Could you check a few things on this model? Use its own coordinates, in mm. Coordinates: 2 decimals unless noted, no trailing zeros. Answer as CSV lines item,"result". Start each with the question number.
Item 1: Suppose I cut it at A-A, the plane z = 378. State how many separate pieces and enclosed holes the cut face has, and give its area (3 significant figures).
Item 2: I'm going to push flat-ended pins straight in: P1, Ø2.5, axis at y = -1.5, z = 150.5, coming from the +X side; P2, Ø1.5, axis at x = -10.5, z = 110.5, coming from the -Y side. Where does each tip first touch, or does it pass through?
Item 3: If I drill on line 1 along X through (y, z) = (7, 64.5); line 2 along Y through (x, z) = (-15, 459); line 3 along Y through (x, z) = (-9.5, 274), over which ranges is the centre line in solid material (lowest first)? Write a range as [from, to].
```python
from build123d import *

# Parameters (mm, degrees)
F0_R     = 2.1
F1_DEPTH = 500


with BuildPart() as f1:
    # F0 (on Top) → F1 (new body)
    with BuildSketch(Plane.XY):
        with BuildLine():
            Line((14.135135, -0.519615), (13.835135, 0))
            Line((13.835135, 0), (14.135135, 0.519615))
            Line((14.135135, 0.519615), (14.135135, 2.93934))
            Line((14.135135, 2.93934), (17.195795, 6))
            Line((17.195795, 6), (18.135135, 6))
            Line((18.135135, 6), (18.135135, 3))
            Line((18.135135, 3), (20.135135, 3))
            Line((20.135135, 3), (20.135135, 9))
            ThreePointArc((20.135135, 9), (19.842242, 9.707107), (19.135135, 10))
            Line((19.135135, 10), (13.135135, 10))
            Line((13.135135, 10), (13.135135, 8))
            Line((13.135135, 8), (16.135135, 8))
            Line((16.135135, 8), (16.135135, 7.06066))
            Line((16.135135, 7.06066), (13.074475, 4))
            Line((13.074475, 4), (10.65475, 4))
            Line((10.65475, 4), (10.135135, 3.7))
            Line((10.135135, 3.7), (9.61552, 4))
            Line((9.61552, 4), (7.195795, 4))
            Line((7.195795, 4), (4.135135, 7.06066))
            Line((4.135135, 7.06066), (4.135135, 8))
            Line((4.135135, 8), (7.135135, 8))
            Line((7.135135, 8), (7.135135, 10))
            Line((7.135135, 10), (-6.864865, 10))
            Line((-6.864865, 10), (-6.864865, 8))
            Line((-6.864865, 8), (-3.864865, 8))
            Line((-3.864865, 8), (-3.864865, 7.06066))
            Line((-3.864865, 7.06066), (-6.925525, 4))
            Line((-6.925525, 4), (-9.34525, 4))
            Line((-9.34525, 4), (-9.864865, 3.7))
            Line((-9.864865, 3.7), (-10.38448, 4))
            Line((-10.38448, 4), (-12.804205, 4))
            Line((-12.804205, 4), (-15.864865, 7.06066))
            Line((-15.864865, 7.06066), (-15.864865, 8))
            Line((-15.864865, 8), (-12.864865, 8))
            Line((-12.864865, 8), (-12.864865, 10))
            Line((-12.864865, 10), (-18.864865, 10))
            ThreePointArc((-18.864865, 10), (-19.571972, 9.707107), (-19.864865, 9))
            Line((-19.864865, 9), (-19.864865, 3))
            Line((-19.864865, 3), (-17.864865, 3))
            Line((-17.864865, 3), (-17.864865, 6))
            Line((-17.864865, 6), (-16.925525, 6))
            Line((-16.925525, 6), (-13.864865, 2.93934))
            Line((-13.864865, 2.93934), (-13.864865, 0.519615))
            Line((-13.864865, 0.519615), (-13.564865, 0))
            Line((-13.564865, 0), (-13.864865, -0.519615))
            Line((-13.864865, -0.519615), (-13.864865, -2.93934))
            Line((-13.864865, -2.93934), (-16.925525, -6))
            Line((-16.925525, -6), (-17.864865, -6))
            Line((-17.864865, -6), (-17.864865, -3))
            Line((-17.864865, -3), (-19.864865, -3))
            Line((-19.864865, -3), (-19.864865, -9))
            ThreePointArc((-19.864865, -9), (-19.571972, -9.707107), (-18.864865, -10))
            Line((-18.864865, -10), (-12.864865, -10))
            Line((-12.864865, -10), (-12.864865, -8))
            Line((-12.864865, -8), (-15.864865, -8))
            Line((-15.864865, -8), (-15.864865, -7.06066))
            Line((-15.864865, -7.06066), (-12.804205, -4))
            Line((-12.804205, -4), (-10.38448, -4))
            Line((-10.38448, -4), (-9.864865, -3.7))
            Line((-9.864865, -3.7), (-9.34525, -4))
            Line((-9.34525, -4), (-6.925525, -4))
            Line((-6.925525, -4), (-3.864865, -7.06066))
            Line((-3.864865, -7.06066), (-3.864865, -8))
            Line((-3.864865, -8), (-6.864865, -8))
            Line((-6.864865, -8), (-6.864865, -10))
            Line((-6.864865, -10), (7.135135, -10))
            Line((7.135135, -10), (7.135135, -8))
            Line((7.135135, -8), (4.135135, -8))
            Line((4.135135, -8), (4.135135, -7.06066))
            Line((4.135135, -7.06066), (7.195795, -4))
            Line((7.195795, -4), (9.61552, -4))
            Line((9.61552, -4), (10.135135, -3.7))
            Line((10.135135, -3.7), (10.65475, -4))
            Line((10.65475, -4), (13.074475, -4))
            Line((13.074475, -4), (16.135135, -7.06066))
            Line((16.135135, -7.06066), (16.135135, -8))
            Line((16.135135, -8), (13.135135, -8))
            Line((13.135135, -8), (13.135135, -10))
            Line((13.135135, -10), (19.135135, -10))
            ThreePointArc((19.135135, -10), (19.842242, -9.707107), (20.135135, -9))
            Line((20.135135, -9), (20.135135, -3))
            Line((20.135135, -3), (18.135135, -3))
            Line((18.135135, -3), (18.135135, -6))
            Line((18.135135, -6), (17.195795, -6))
            Line((17.195795, -6), (14.135135, -2.93934))
            Line((14.135135, -2.93934), (14.135135, -0.519615))
        make_face()
        with Locations((-9.864865, 0)):
            Circle(F0_R, mode=Mode.SUBTRACT)
        Polygon((6.435135, 0), (6.135135, -0.519615), (6.135135, -2.93934), (3.074475, -6), (2.013815, -7.06066), (2.013815, -8), (-1.743545, -8), (-1.743545, -7.06066), (-2.804205, -6), (-5.864865, -2.93934), (-5.864865, -0.519615), (-6.164865, 0), (-5.864865, 0.519615), (-5.864865, 2.93934), (-2.804205, 6), (-1.743545, 7.06066), (-1.743545, 8), (2.013815, 8), (2.013815, 7.06066), (3.074475, 6), (6.135135, 2.93934), (6.135135, 0.519615), align=None, mode=Mode.SUBTRACT)
        with Locations((10.135135, 0)):
            Circle(F0_R, mode=Mode.SUBTRACT)
    extrude(amount=F1_DEPTH)


solid = f1.part
```
Ans:
1,separate pieces,"1"
1,enclosed holes,"3"
1,area,"324 mm^2"
2,P1,"stops at x = 14.14"
2,P2,"stops at y = -4"
3,line 1,"x = [-19.86, -15.8], [-3.93, -1.8], [2.07, 4.2], [16.07, 20.14]"
3,line 2,"y = [-10, -8], [-6.2, -4.07], [4.07, 6.2], [8, 10]"
3,line 3,"y = [-3.91, -2.07], [2.07, 3.91]"
